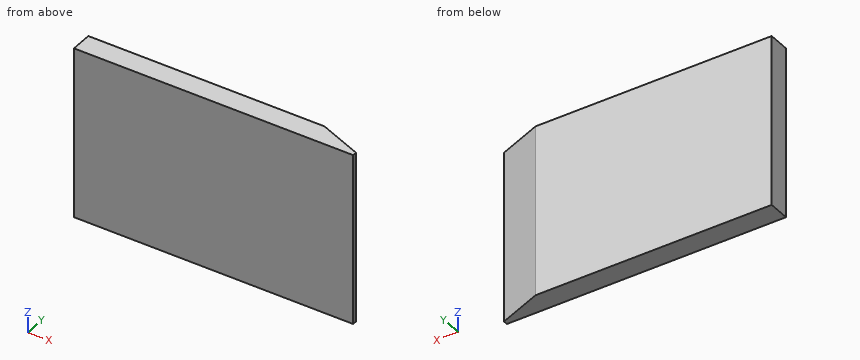
from build123d import *

# Parameters (mm, degrees)
SKETCH1_W           = 130
SKETCH1_H           = 80
BOSS_EXTRUDE1_DEPTH = 10
CUT_EXTRUDE1_DEPTH  = 81


with BuildPart() as part:
    # Sketch1 → Boss-Extrude1 (new body)
    with BuildSketch(Plane(origin=(0, 0, 0), x_dir=(1, 0, 0), z_dir=(0, 1, 0))):
        Rectangle(SKETCH1_W, SKETCH1_H)
    extrude(amount=BOSS_EXTRUDE1_DEPTH)

    # Sketch2 → Cut-Extrude1 (cut, through all)
    with BuildSketch(Plane.XY.offset(40)):
        Polygon((65, 2), (45, 10), (65, 10), align=None)
    extrude(amount=-CUT_EXTRUDE1_DEPTH, mode=Mode.SUBTRACT)


solid = part.part
Read the model definition and answer for the solid it produces. Units are mm, in the model's axes. Give positions to 0.01 mm unless a question says otherwise; leave off trailing zeros. Write each loop counter-clockwise with the first axis right and the second up, starting at its lowest first coordinate (ties: lowest second). Pieces come first, ordered by that corner, then holes. Notation, with made-up numbers: (72, -38.5) - (97, -38.5) arc R30 ccw to (97, 0.5) - close; hole circle Ø4 at (-25, -12). An arc over 180 degrees is marked (long way). Use CSV: the item, a comma, the result in double quotes. Start each with the question number.
Item 1: The part is cut by section B-B, the plane y = 7.5. Give the vertices of the cut face in (x, z), and give its area (3 significant figures).
Item 2: Consider line 1 (Y direction, x = 52.5, z = -19.5); line 2 (X direction, y = 9, z = 34.5). Determine where each line is inside the solid, lowest interval first.
Item 3: The part is cut by section A-A, the plane z = 14.5. Give the vertices of the cut face in (x, y), and give its area (3 significant figures).
Taken from the geometry:
1,outline,"(-65, -40) - (51.25, -40) - (51.25, 40) - (-65, 40) - close"
1,area,"9,300 mm2"
2,line 1,"0 to 7"
2,line 2,"-65 to 47.5"
3,outline,"(-65, 0) - (65, 0) - (65, 2) - (45, 10) - (-65, 10) - close"
3,area,"1,220 mm2"
